Work out the finished part from the listing and answer in its coordinate system (mm). A direction names the side the tool comes from. Give positions to 0.01 mm unless a question says otherwise; leave off trailing zeros. Loops run counter-clockwise (first coordinate to the right, second up) from the corner with the lowest first, then second, coordinate; pieces in that order, holes last.
Autodesk Fusion 360 part; units mm, degrees
sketch "Sketch1" plane through (0, 0, 0) normal (0, 1, 0) x (1, 0, 0)
  line L0 (0, 0) -> (20, 0)
  line L1 (0, -20) -> (0, 0)
  line L2 (20, 0) -> (20, -3)
  line L3 (0, -20) -> (3, -20)
  line L4 (3, -20) -> (20, -3)
extrude "Extrude1" add sketch "Sketch1" along normal blind 15
sketch "Sketch2" plane through (0, 0, 20) normal (0, 0, 1) x (1, 0, 0)
  line L0 (0, 0) -> (3, 0)
  line L1 (3, 0) -> (3, 15)
  line L2 (3, 15) -> (0, 15)
  line L3 (0, 15) -> (0, 0)
  line L4 (2, 14) -> (20, 14)
  line L5 (20, 14) -> (20, 1)
  line L6 (20, 1) -> (2, 1)
  line L7 (2, 1) -> (2, 14)
extrude "Extrude2" cut sketch "Sketch2" against normal blind 18 contours L1 L4 L6 L7 | L1 L4 L5 L6
sketch "Sketch3" plane through (0, 0, 2) normal (0, 0, 1) x (1, 0, 0)
  line L0 (2, 1) -> (20, 1)
  line L1 (20, 1) -> (20, 14)
  line L2 (20, 14) -> (2, 14)
  line L3 (2, 14) -> (2, 1)
  arc A0 (10.0508, 9.7) -> (10.0508, 5.3) centre (10.05, 7.5) ccw
  arc A1 (11.95, 5.3) -> (11.95, 9.7) centre (11.95, 7.5) ccw
  line L4 (10.0508, 9.7) -> (11.95, 9.7)
  line L5 (10.0508, 5.3) -> (11.95, 5.3)
  dimension "d5" = 4.4
  dimension "d6" = 4.4
  dimension "d8" = 1.9
  dimension "d9" = 8.05
revolve "Revolve1" cut sketch "Sketch3" angle 360 about axis through (2, 14, 2) along (0, -1, 0) contours A0 A1 L4 L5
equation "d8 = 6.3 mm - 4.4 mm"
Item 1: Determine the mould class of faces 1 (the face through (1, 7, 20)), 2 (the face through (9, 1, 9)), 3 (the face through (8, 15, 8)) for opening direction Y: released by +Y, released by -Y, zero draft, split by the parting line, or undercut.
Item 2: Find section A-A, the plane x = 11. Write down the section's boundary in (y, z).
Item 3: For faces 4 (the face through (1, 9.7, 11)), 5 (the face through (8, 0, 8)), 6 (the face through (2, 10, 11)), determine the directions among +Z, -Z, +X, -X, +Y, -Y from which every point of the face is accessible in a straight line to the end or side of a thin tool.
Item 4: Find section D-D, the plane x = 17.25. Write down the section's boundary in (y, z), plus the area to 3 significant figures.
Item 5: A flat-ended cylindrical pin translates along its axis: pin 1 Ø8 at (x, y) = (8, 9) entering from +Z. Find the tip coordinate at first contact, or state that the pin passes through.
Item 6: Find section C-C, the plane y = 8.5. Write down the section's boundary in (x, z), plus the area to 3 significant figures.
Item 7: Find section B-B, the plane z = 10.75. Write down the section's boundary in (x, y), plus the area to 3 significant figures.
Item 8: Consider line 1 (Y direction, x = 4.75, z = 10.25); line 2 (Z direction, x = 6.75, y = 9.25). Determine where each line is inside the solid, lowest interval first.
Ans:
1. face 1: zero draft
1. face 2: undercut
1. face 3: released by +Y
2. outline: (0, 0) - (5.3, 0) - (5.3, 2) - (1, 2) - (1, 12) - (0, 12) - close; (9.7, 0) - (15, 0) - (15, 12) - (14, 12) - (14, 2) - (9.7, 2) - close
3. face 4: +X, -X
3. face 5: +Z, -Z, +X, -X, -Y
3. face 6: +Z, +X
4. outline: (0, 0) - (15, 0) - (15, 5.75) - (14, 5.75) - (14, 2) - (1, 2) - (1, 5.75) - (0, 5.75) - close
4. area: 37.5 mm2
5. pin 1: stops at z = 2
6. outline: (0, 0) - (7.75, 0) arc R6.09 ccw to (8.09, 2) - (2, 2) - (2, 8.09) arc R6.09 ccw to (0, 7.75) - close; (0, 13.74) arc R11.91 cw to (2, 13.91) - (2, 20) - (0, 20) - close; (13.74, 0) - (20, 0) - (20, 2) - (13.91, 2) arc R11.91 cw to start
6. area: 52.5 mm2
7. outline: (0, 0) - (12.25, 0) - (12.25, 1) - (2, 1) - (2, 5.3) - (0, 5.3) - close; (0, 9.7) - (2, 9.7) - (2, 14) - (12.25, 14) - (12.25, 15) - (0, 15) - close
7. area: 41.7 mm2
8. line 1: y = 0 to 1, 14 to 15
8. line 2: z = 0 to 2
